```python
from build123d import *

# Parameters (mm, degrees)
F1_DEPTH = 5
F3_DEPTH = 5


# Not quite as in the source:
# - ends of sketch curves that miss each other by under 0.0002 mm in the source are joined
# - a feature names something its author has since deleted; it is built from what else it names


with BuildPart() as f1:
    # F0 (on Top) → F1 (new body)
    with BuildSketch(Plane.XY):
        with BuildLine():
            Line((0, 29.2999204248), (0, 0))
            Line((0, 0), (34.4714387385, 0))
            Line((34.4714387385, 0), (34.4714387385, 16.3473710418))
            ThreePointArc((34.4714387385, 16.3473710418), (32.5790927131, 15.1300794804), (32.2559916738, 17.3568210333))
            ThreePointArc((32.2559916738, 17.3568210333), (15.182844974, 14.8438668457), (5.7578901922, 29.2999210911))
            ThreePointArc((5.7578901922, 29.2999210911), (2.8789043427, 26.4210160822), (0, 29.2999204248))
        make_face()
        with BuildLine():
            ThreePointArc((5.7577396052, 29.3198639813), (2.8689325046, 32.1788074974), (0, 29.2999204248))
            ThreePointArc((0, 29.2999204248), (2.8789043427, 26.4210160822), (5.7578086853, 29.2999204248))
            ThreePointArc((5.7578086853, 29.2999204248), (5.7578117914, 29.3098925127), (5.7577396052, 29.3198639813))
        make_face()
        with BuildLine():
            ThreePointArc((32.2559916738, 17.3568210333), (32.5790927131, 15.1300794804), (34.4714387385, 16.3473710418))
            ThreePointArc((34.4714387385, 16.3473710418), (33.6883902233, 17.5646626032), (32.2559916738, 17.3568210333))
        make_face()
    extrude(amount=F1_DEPTH)

    # F2 (on face) → F3 (join)
    with BuildSketch(Plane.XY.offset(5)):
        with BuildLine():
            ThreePointArc((34.4714387385, 16.3473710418), (33.6883902233, 17.5646626032), (32.2559916738, 17.3568210333))
            ThreePointArc((32.2559916738, 17.3568210333), (15.182844974, 14.8438668457), (5.7578901922, 29.2999210911))
            ThreePointArc((5.7578901922, 29.2999210911), (5.757811792, 29.3098923335), (5.7577396052, 29.3198639813))
            ThreePointArc((5.7577396052, 29.3198639813), (2.8689325046, 32.1788074974), (0, 29.2999204248))
            Line((0, 29.2999204248), (0, 0))
            Line((0, 0), (34.4714387385, 0))
            Line((34.4714387385, 0), (34.4714387385, 16.3473710418))
        make_face()
    extrude(amount=-F3_DEPTH)


solid = f1.part
```
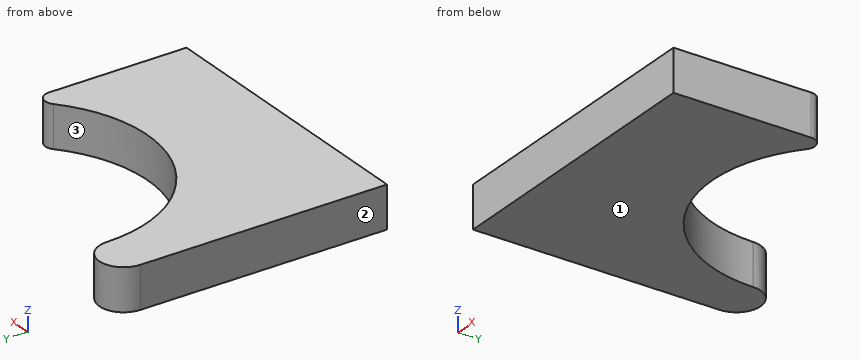
Could you check a few things on this model? Use its own coordinates, in mm. Face numbers are marked on the shaded views. Give positions to 0.01 mm unless a question says otherwise; leave off trailing zeros. Loops run counter-clockwise (first coordinate to the right, second up) from the corner with the lowest first, then second, coordinate; pieces in that order, holes last. Notation, with made-up numbers: (50.5, 43.25) - (106.5, 43.25) arc R20 ccw to (106.5, 74.25) - close; hole circle Ø6 at (70, -3). An arc over 180 degrees is marked (long way). Answer in a Markdown table with one row per item. Add a question column.
Q1. If we section it at C-C (x = 27): List the corners of the cut face in (y, z) for me, plus the area to 3 significant figures.
Q2. Please list where these lines run through material, in increasing order: L1, parallel to X at y = 17, z = 4.55; L2, parallel to Y at x = 33, z = 2.25; L3, parallel to X at y = 26, z = 0.7. Write a range as from..to.
Q3. If we section it at B-B (y = 24.5): List the corners of the cut face in (x, z) for me.
Q4. We'd pull the mould along X, two halves only. Please class the marked faces 1, 2 and 3: +X half, -X half, draft (parallel to the pull), parting line (faces both ways), or undercut.
Q5. For pin 1 (2 mm diameter, centred on x = 15, z = 4, fed in from -Y), with a flat end and sliding along its axis, tell me the tip position at first contact or that it passes through.
The answers:
| question | item | result |
|---|---|---|
| 1 | outline | (0, 0) - (14.31, 0) - (14.31, 5) - (0, 5) - close |
| 1 | area | 71.6 mm^2 |
| 2 | L1 | x = 0..11.68, 31.83..34.3 |
| 2 | L2 | y = 0..17.68 |
| 2 | L3 | x = 0..6.13 |
| 3 | outline | (0, 0) - (6.54, 0) - (6.54, 5) - (0, 5) - close |
| 4 | face 1 | draft |
| 4 | face 2 | -X half |
| 4 | face 3 | undercut |
| 5 | pin 1 | stops at y = 0 |
